Input: part model. Units: mm. Frame: model coordinates. Face numbers are marked on the shaded views. A direction names the side the tool comes from. Round coordinates to 2 decimals unless told otherwise and drop trailing zeros. Loops run counter-clockwise (first coordinate to the right, second up) from the corner with the lowest first, then second, coordinate; pieces in that order, holes last. Notation, with made-up numbers: (44.25, 88) - (102.25, 88) arc R28 ccw to (102.25, 116) - close; hole circle Ø11 at (56, 36.25). An arc over 180 degrees is marked (long way). One line per question, with ' | ' between items. Start each with the question number.
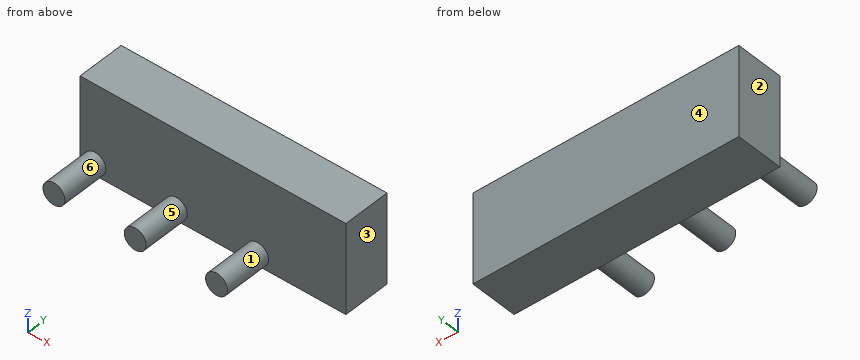
from build123d import *

# Parameters (mm, degrees)
F0_W     = 142.000898
F0_H     = 48.036786
F1_DEPTH = 25.4
F2_R     = 5.849573
F3_DEPTH = 25.4


with BuildPart() as f1:
    # F0 (on Front) → F1 (new body)
    with BuildSketch(Plane.XZ):
        with Locations((1.806505, 27.979008)):
            Rectangle(F0_W, F0_H)
    extrude(amount=F1_DEPTH)

    # F2 (on face) → F3 (join)
    with BuildSketch(Plane.XZ.offset(25.4)):
        with Locations((-61.215024, 10.251221)):
            Circle(F2_R)
        with Locations((-17.781024, 10.251221)):
            Circle(F2_R)
        with Locations((25.652976, 10.251221)):
            Circle(F2_R)
    extrude(amount=F3_DEPTH)


solid = f1.part
(1) Section C-C, the plane y = -41.5. Output: boundary loops of the cut face in (x, z), plus the area to 3 significant figures.
(2) Line query: line 1 along X through (y, z) = (-34, 6); line 2 along X through (y, z) = (-35.5, 15); line 3 along Y through (x, z) = (-11.5, 40). Output: solid intervals per line, ascending. Write a range as from..to.
(3) Pin query (flat end, axial travel): P1, Ø3, axis at x = -42.5, z = 32.5, coming from the -Y side; P2, Ø12, axis at y = -34.5, z = 43, coming from the -X side. Return the tip coordinate at first contact, or that it passes through.
(4) Section D-D, the plane x = 44. Output: boundary loops of the cut face in (y, z), plus the area to 3 significant figures.
(5) Section B-B, the plane z = 42. Output: boundary loops of the cut face in (x, y).
(6) Section A-A, the plane x = -20. Output: boundary loops of the cut face in (y, z), plus the area to 3 significant figures.
(7) Pull-direction query (X, two-part tool) for the marked faces 3, 4, 5 and 6; classes: released by +X, released by -X, zero draft, split by the parting line, or undercut.
(8) Reachability of the marked faces 1 and 2 from +Z, -Z, +X, -X, +Y, -Y: full face, straight path, thin tool, end or side. Return the list, or none.
Derived:
1) outline: circle Ø11.7 at (-61.22, 10.25); circle Ø11.7 at (-17.78, 10.25); circle Ø11.7 at (25.65, 10.25) | area: 322 mm²
2) line 1: x = -65.23..-57.2, -21.8..-13.76, 21.63..29.67 | line 2: x = -64.63..-57.8, -21.2..-14.37, 22.24..29.07 | line 3: y = -25.4..0
3) P1: stops at y = -25.4 | P2: passes through
4) outline: (-25.4, 3.96) - (0, 3.96) - (0, 52) - (-25.4, 52) - close | area: 1,220 mm²
5) outline: (-69.19, -25.4) - (72.81, -25.4) - (72.81, 0) - (-69.19, 0) - close
6) outline: (-50.8, 4.84) - (-25.4, 4.84) - (-25.4, 3.96) - (0, 3.96) - (0, 52) - (-25.4, 52) - (-25.4, 15.66) - (-50.8, 15.66) - close | area: 1,500 mm²
7) face 3: released by +X | face 4: zero draft | face 5: undercut | face 6: undercut
8) face 1: -Y | face 2: +Z, -Z, -X, +Y, -Y
